The model under review builds one solid part; all positions refer to its coordinate system, in mm. A direction names the side the tool comes from. Give positions to 0.01 mm unless a question says otherwise; leave off trailing zeros. Loops run counter-clockwise (first coordinate to the right, second up) from the corner with the lowest first, then second, coordinate; pieces in that order, holes last. Notation, with made-up numbers: (36.5, 16) - (46.5, 16) arc R26 cw to (46.5, 42) - close; hole circle Ø3 at (-29.5, 32.25). An arc over 180 degrees is marked (long way). Return JSON: item names as keys, results as strings. Group by question number.
from build123d import *

# Parameters (mm, degrees)
SKETCH1_W           = 46
SKETCH1_H           = 70
BOSS_EXTRUDE1_DEPTH = 2
BOSS_EXTRUDE2_DEPTH = 16.3
SKETCH3_W           = 23.1
SKETCH3_H           = 12.6
CUT_EXTRUDE1_DEPTH  = 45.940961271
SKETCH4_W           = 34
SKETCH4_H           = 14.8
BOSS_EXTRUDE3_DEPTH = 11.125
BOSS_EXTRUDE4_DEPTH = 12.5
SKETCH7_W           = 6.36
SKETCH7_H           = 14.8
CUT_EXTRUDE2_DEPTH  = 9.125
SKETCH8_W           = 13
SKETCH8_H           = 12.5
SKETCH8_R           = 0.95
BOSS_EXTRUDE5_DEPTH = 2.52
BOSS_EXTRUDE6_DEPTH = 27.64
SKETCH10_W          = 7
SKETCH10_H          = 4.8
CUT_EXTRUDE3_DEPTH  = 12.5
SKETCH11_R          = 3.5
CUT_EXTRUDE4_DEPTH  = 10
SKETCH12_R          = 1.1
CUT_EXTRUDE5_DEPTH  = 8
CUT_EXTRUDE6_DEPTH  = 1.8
SKETCH14_R          = 1.1
CUT_EXTRUDE7_DEPTH  = 5
CUT_EXTRUDE8_DEPTH  = 2


with BuildPart() as part:
    # Sketch1 → Boss-Extrude1 (new body)
    with BuildSketch(Plane(origin=(0, 0, 0), x_dir=(1, 0, 0), z_dir=(0, 1, 0))):
        Rectangle(SKETCH1_W, SKETCH1_H)
    extrude(amount=BOSS_EXTRUDE1_DEPTH)

    # Sketch2 → Boss-Extrude2 (add)
    with BuildSketch(Plane(origin=(0, 2, 0), x_dir=(1, 0, 0), z_dir=(0, 1, 0))):
        Polygon((16.94, 22.4), (16.94, 35), (21.74, 35), (21.74, 20.9), (-10.96, 20.9), (-10.96, 35), (-6.16, 35), (-6.16, 22.4), align=None)
    extrude(amount=BOSS_EXTRUDE2_DEPTH)

    # Sketch3 → Cut-Extrude1 (cut, through all)
    with BuildSketch(Plane(origin=(0, 2, 0), x_dir=(1, 0, 0), z_dir=(0, 1, 0))):
        with Locations((5.39, 28.7)):
            Rectangle(SKETCH3_W, SKETCH3_H)
    extrude(amount=-CUT_EXTRUDE1_DEPTH, mode=Mode.SUBTRACT)

    # Sketch4 → Boss-Extrude3 (add)
    with BuildSketch(Plane.XZ):
        with Locations((0, 27.6)):
            Rectangle(SKETCH4_W, SKETCH4_H)
    extrude(amount=-BOSS_EXTRUDE3_DEPTH)

    # Sketch5 → Boss-Extrude4 (add)
    with BuildSketch(Plane(origin=(0, 11.125, 0), x_dir=(1, 0, 0), z_dir=(0, 1, 0))):
        Polygon((-14.48, -35), (-17, -35), (-17, -20.2), (10.64, -20.2), (10.64, -35), (8.12, -35), (8.12, -25), (-14.48, -25), align=None)
    extrude(amount=BOSS_EXTRUDE4_DEPTH)

    # Sketch7 → Cut-Extrude2 (cut)
    with BuildSketch(Plane(origin=(0, 11.125, 0), x_dir=(1, 0, 0), z_dir=(0, 1, 0))):
        with Locations((13.82, -27.6)):
            Rectangle(SKETCH7_W, SKETCH7_H)
    extrude(amount=-CUT_EXTRUDE2_DEPTH, mode=Mode.SUBTRACT)

    # Sketch8 → Boss-Extrude5 (add)
    with BuildSketch(Plane(origin=(-14.48, 0, 0), x_dir=(0, 0, -1), z_dir=(1, 0, 0))):
        with Locations((-41.5, 17.375)):
            Rectangle(SKETCH8_W, SKETCH8_H)
        with Locations((-41.939, 17.375)):
            Circle(SKETCH8_R, mode=Mode.SUBTRACT)
    extrude(amount=-BOSS_EXTRUDE5_DEPTH)

    # Sketch9 → Boss-Extrude6 (add)
    with BuildSketch(Plane.ZY.offset(17)):
        Polygon((48, 11.125), (35, 0), (35, 11.125), align=None)
    extrude(amount=-BOSS_EXTRUDE6_DEPTH)

    # Sketch10 → Cut-Extrude3 (cut)
    with BuildSketch(Plane(origin=(0, 23.625, 0), x_dir=(1, 0, 0), z_dir=(0, 1, 0))):
        with Locations((7.14, -22.6)):
            Rectangle(SKETCH10_W, SKETCH10_H)
    extrude(amount=-CUT_EXTRUDE3_DEPTH, mode=Mode.SUBTRACT)

    # Sketch11 → Cut-Extrude4 (cut)
    with BuildSketch(Plane(origin=(10.64, 0, 0), x_dir=(0, 0, -1), z_dir=(1, 0, 0))):
        with Locations((-36.06, 17.375)):
            Circle(SKETCH11_R)
    extrude(amount=-CUT_EXTRUDE4_DEPTH, mode=Mode.SUBTRACT)

    # Sketch12 → Cut-Extrude5 (cut)
    with BuildSketch(Plane(origin=(3.64, 0, 0), x_dir=(0, 0, -1), z_dir=(1, 0, 0))):
        with Locations((-22.62, 17.375)):
            Circle(SKETCH12_R)
    extrude(amount=-CUT_EXTRUDE5_DEPTH, mode=Mode.SUBTRACT)

    # Sketch13 → Cut-Extrude6 (cut)
    with BuildSketch(Plane(origin=(1.64, 0, 0), x_dir=(0, 0, -1), z_dir=(1, 0, 0))):
        Polygon((-21.494166975, 19.325), (-19.2, 19.325), (-19.2, 15.425), (-21.494166975, 15.425), (-23.745833025, 15.425), (-24.87166605, 17.375), (-23.745833025, 19.325), align=None)
    extrude(amount=-CUT_EXTRUDE6_DEPTH, mode=Mode.SUBTRACT)

    # Sketch14 → Cut-Extrude7 (cut)
    with BuildSketch(Plane(origin=(0, 18.3, 0), x_dir=(1, 0, 0), z_dir=(0, 1, 0))):
        with Locations(Location((-8.46, 28.65, 0), (0, 0, 270))):
            Circle(SKETCH14_R)
        with Locations(Location((19.24, 28.65, 0), (0, 0, 270))):
            Circle(SKETCH14_R)
    extrude(amount=-CUT_EXTRUDE7_DEPTH, mode=Mode.SUBTRACT)

    # Sketch15 → Cut-Extrude8 (cut)
    with BuildSketch(Plane(origin=(0, 16.3, 0), x_dir=(1, 0, 0), z_dir=(0, 1, 0))):
        Polygon((18.085299462, 30.65), (16.94, 30.65), (16.94, 26.65), (18.085299462, 26.65), (20.394700538, 26.65), (21.549401077, 28.65), (20.394700538, 30.65), align=None)
        Polygon((-6.16, 26.65), (-7.305299462, 26.65), (-9.614700538, 26.65), (-10.769401077, 28.65), (-9.614700538, 30.65), (-7.305299462, 30.65), (-6.16, 30.65), align=None)
    extrude(amount=-CUT_EXTRUDE8_DEPTH, mode=Mode.SUBTRACT)


solid = part.part
Item 1: For P1, Ø6, axis at y = 6, z = -17, coming from the -X side; P2, Ø2, axis at y = 5, z = 19.5, coming from the -X side; P3, Ø1, axis at x = 1.5, z = 34.5, coming from the +Y side (3 decimals); P4, Ø2, axis at x = -8.5, y = 15, coming from the +Z side, all flat-tipped, find the tip position at first contact; note any pin that passes through.
Item 2: For L1, parallel to X at y = 16.75, z = -28.65; L2, parallel to X at y = 13.5, z = 34; L3, parallel to X at y = 10, z = -26, list the stretches that pass through material, from the lowest coordinate up. Write a range as from..to.
Item 3: Take a section at C-C (x = 19.24). State the section outline as (y, z) points, then the cut area to 3 significant figures.
Item 4: Take a section at D-D (z = -2.5). State the section outline as (x, y) points.
Item 5: Take a section at B-B (y = 5.25). State the section outline as (x, z) points, then the cut area to 3 significant figures.
Item 6: Tool access review of faces 4 (the face through (-6.16, 9, -29)), 5 (the face through (0.753, 16.386, 24.301)), 6 (the face through (9, 17, 25)): name each direction out of +Z, -Z, +X, -X, +Y, -Y from which nothing blocks a thin tool from reaching the whole face with its end or side.
Item 7: Take a section at A-A (x = -3.5). State the section outline as (y, z) points (3 decimals).
Item 8: Mouldability with a two-part tool opening along Z and no side actions: class faces 1 (the face through (3.64, 19, 23)), 2 (the face through (19, 15, -30.65)), 3 (the face through (-9, 7, -35)) as +Z half, -Z half, draft (parallel to the pull), parting line (faces both ways), or undercut.
Check sheet entries:
{
 "1": {"P1": "passes through", "P2": "stops at x = -17", "P3": "stops at y = 11.125", "P4": "stops at z = 25"},
 "2": {"L1": "x = -10.96..-9.56, -7.36..-6.16, 16.94..18.14, 20.34..21.74", "L2": "x = -17..-14.48, 8.12..10.64", "L3": "x = -10.96..-6.16, 16.94..21.74"},
 "3": {"outline": "(0, -35) - (18.3, -35) - (18.3, -29.75) - (16.3, -29.75) - (16.3, -30.65) - (14.3, -30.65) - (14.3, -29.75) - (13.3, -29.75) - (13.3, -27.55) - (14.3, -27.55) - (14.3, -26.65) - (16.3, -26.65) - (16.3, -27.55) - (18.3, -27.55) - (18.3, -20.9) - (2, -20.9) - (2, 35) - (0, 35) - close", "area": "355 mm^2"},
 "4": {"outline": "(-23, 0) - (23, 0) - (23, 2) - (-23, 2) - close"},
 "5": {"outline": "(-17, 20.2) - (10.64, 20.2) - (10.64, 41.13) - (-17, 41.13) - close; (-10.96, -35) - (-6.16, -35) - (-6.16, -22.4) - (16.94, -22.4) - (16.94, -35) - (21.74, -35) - (21.74, -20.9) - (-10.96, -20.9) - close", "area": "749 mm^2"},
 "6": {"face 4": "-Z, +Y, -Y", "face 5": "none", "face 6": "+X, +Y"},
 "7": {"outline": "(0, -22.4) - (18.3, -22.4) - (18.3, -20.9) - (2, -20.9) - (2, 20.2) - (23.625, 20.2) - (23.625, 25) - (11.125, 25) - (11.125, 48) - (0, 35) - close; hole circle Ø2.2 at (17.375, 22.62)"},
 "8": {"face 1": "draft", "face 2": "undercut", "face 3": "-Z half"}
}
